Verification items for this drawing (mm, ordinates from the low corner). Round coordinates to 2 decimals unless told otherwise and drop trailing zeros. Loops run counter-clockwise (first coordinate to the right, second up) from the corner with the lowest first, then second, coordinate; pieces in that order, holes last. Notation, with made-up numbers: M 56,33.5 L 91,33.5 A34 cw 91,69.5 Z; hole C 19.25,45 d6. An arc over 180 degrees is marked long. Write item = value, one per line. Start each with the question number.
(1) Cross-section at A-A on y = 6.5. Record the boundary of the cut face in (x, z), plus the area to 3 significant figures.
(2) Mould release check, pull along X, two halves, no side actions. Record for the marked faces 1, 2 and 3: pulls with the +X half, pulls with the -X half, needs draft (parallel to the pull), parting line crosses it, or undercut.
(3) Go/stop test with flat-tipped pins: P1, Ø2, axis at x = 9, y = 9.5, coming from the +Z side; P2, Ø2, axis at y = 4, z = 1.5, coming from the +X side; P3, Ø3, axis at y = 2, z = 2, coming from the -X side. Record where each tip stops, or that it passes through.
(4) Scan lines: L1, parallel to Y at x = 6.5, z = 1.35; L2, parallel to X at y = 5.5, z = 3.35; L3, parallel to X at y = 7.5, z = 4.6. Record each from-to range of solid material in increasing order. Write a range as from..to.
(5) Cross-section at B-B on z = 3.1. Record the boundary of the cut face in (x, y).
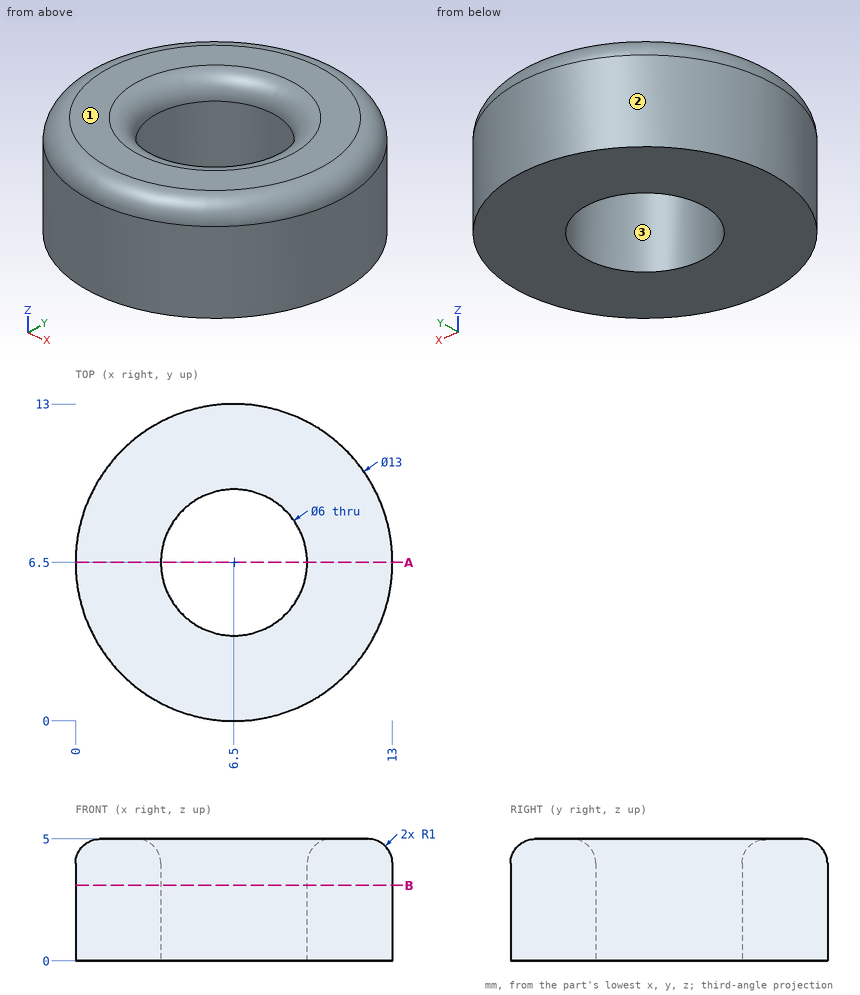
Result:
q1.outline = M 0,0 L 3.5,0 L 3.5,4 A1 ccw 2.5,5 L 1,5 A1 ccw 0,4 Z; M 9.5,0 L 13,0 L 13,4 A1 ccw 12,5 L 10.5,5 A1 ccw 9.5,4 Z
q1.area = 34.1 mm^2
q2.face_1 = needs draft
q2.face_2 = parting line crosses it
q2.face_3 = undercut
q3.P1 = 5
q3.P2 = 12.82
q3.P3 = 0.73
q4.L1 = 0..3.5, 9.5..13
q4.L2 = 0.08..3.67, 9.33..12.92
q4.L3 = 0.28..3.46, 9.54..12.72
q5.outline = C 6.5,6.5 d13; hole C 6.5,6.5 d6
